```python
from build123d import *

# Parameters (mm, degrees)
SKETCH4_W           = 17
SKETCH4_H           = 67
BOSS_EXTRUDE1_DEPTH = 19.5
FILLET1_R           = 1.5
SKETCH5_W           = 13
SKETCH5_H           = 24.5
CUT_EXTRUDE1_DEPTH  = 17.5
SKETCH6_W           = 5.5
SKETCH6_H           = 5.6
CUT_EXTRUDE2_DEPTH  = 12.7
FILLET2_R           = 1
SKETCH7_R           = 1
CUT_EXTRUDE3_DEPTH  = 337.829426821
SKETCH8_W           = 9.5
SKETCH8_H           = 4.5
CUT_EXTRUDE4_DEPTH  = 5
SKETCH9_W           = 8.343526146
SKETCH9_H           = 4.5
CUT_EXTRUDE5_DEPTH  = 5


with BuildPart() as part:
    # Sketch4 → Boss-Extrude1 (new body)
    with BuildSketch(Plane.XY.offset(30)):
        with Locations((-184.236990356, 242.047210693)):
            Rectangle(SKETCH4_W, SKETCH4_H)
    extrude(amount=BOSS_EXTRUDE1_DEPTH)

    # Fillet1
    fillet1_edges = [part.edges().sort_by_distance(p)[0] for p in [
        (-192.736990356, 275.547210693, 39.75),
        (-175.736990356, 275.547210693, 39.75),
        (-175.736990356, 208.547210693, 39.75),
        (-192.736990356, 208.547210693, 39.75),
    ]]
    fillet(fillet1_edges, radius=FILLET1_R)

    # Sketch5 → Cut-Extrude1 (cut)
    with BuildSketch(Plane.XY.offset(49.5)):
        with Locations((-184.236990356, 259.497210693)):
            Rectangle(SKETCH5_W, SKETCH5_H)
        with Locations((-184.236990356, 225.797210693)):
            Rectangle(SKETCH5_W, SKETCH5_H)
    extrude(amount=-CUT_EXTRUDE1_DEPTH, mode=Mode.SUBTRACT)

    # Sketch6 → Cut-Extrude2 (cut)
    with BuildSketch(Plane.XY.offset(49.5)):
        with Locations((-189.986990356, 242.647210693)):
            Rectangle(SKETCH6_W, SKETCH6_H)
        with Locations((-178.486990356, 242.647210693)):
            Rectangle(SKETCH6_W, SKETCH6_H)
    extrude(amount=-CUT_EXTRUDE2_DEPTH, mode=Mode.SUBTRACT)

    # Fillet2
    fillet2_edges = [part.edges().sort_by_distance(p)[0] for p in [
        (-192.736990356, 239.847210693, 43.15),
        (-192.736990356, 245.447210693, 43.15),
        (-175.736990356, 245.447210693, 43.15),
        (-175.736990356, 239.847210693, 43.15),
    ]]
    fillet(fillet2_edges, radius=FILLET2_R)

    # Sketch7 → Cut-Extrude3 (cut, through all)
    with BuildSketch(Plane.XY.offset(49.5)):
        with Locations((-184.236990356, 273.547210693)):
            Circle(SKETCH7_R)
        with Locations((-184.236990356, 210.747210693)):
            Circle(SKETCH7_R)
        with Locations((-184.236990356, 245.247210693)):
            Circle(SKETCH7_R)
        with Locations((-184.236990356, 239.247210693)):
            Circle(SKETCH7_R)
    extrude(amount=-CUT_EXTRUDE3_DEPTH, mode=Mode.SUBTRACT)

    # Sketch8 → Cut-Extrude4 (cut)
    with BuildSketch(Plane(origin=(0, 208.547210693, 0), x_dir=(-1, 0, 0), z_dir=(0, -1, 0))):
        with Locations((184.186990356, -34.25)):
            Rectangle(SKETCH8_W, SKETCH8_H)
    extrude(amount=-CUT_EXTRUDE4_DEPTH, mode=Mode.SUBTRACT)

    # Sketch9 → Cut-Extrude5 (cut)
    with BuildSketch(Plane(origin=(0, 275.547210693, 0), x_dir=(1, 0, 0), z_dir=(0, 1, 0))):
        with Locations((-183.608753429, -34.25)):
            Rectangle(SKETCH9_W, SKETCH9_H)
    extrude(amount=-CUT_EXTRUDE5_DEPTH, mode=Mode.SUBTRACT)


solid = part.part
```
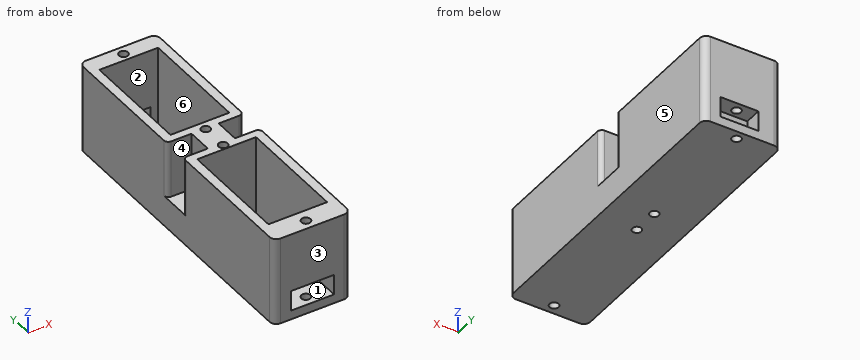
Source: CAD feature listing. Evaluate the final solid. Frame: model axes, mm. Face numbers are marked on the shaded views. A direction names the side the tool comes from. Give positions to 0.01 mm unless a question says otherwise; leave off trailing zeros. Order: outer loops, then holes, each group sorted by start corner. A loop starts at its lowest first (then second) coordinate and runs counter-clockwise, first axis right, second up.
(1) Contact query for flat-ended pins moving along their axis: P1, Ø2.5, axis at x = -184.24, y = 273.55, coming from the -Z side; P2, Ø6.5, axis at x = -182.5, y = 230.5, coming from the +Z side. Output: stop coordinate, or through.
(2) Section query C-C (y = 256). Return the cut outline in (x, z).
(3) Pull-direction query (X, two-part tool) for the marked faces 4, 5 and 6; classes: +X half, -X half, draft (parallel to the pull), parting line (faces both ways), or undercut.
(4) Section query B-B (z = 35.25). Return the cut outline in (x, y).
(5) Access query for the marked faces 1, 2 and 3. Directions: +Z, -Z, +X, -X, +Y, -Y. A direction counts if a zero-diameter tool reaches every point of the face in a straight line with its end or side. Return the directions, or none.
(6) Material intervals for line 1 along Y through (x, z) = (-178.75, 47); line 2 along Y through (x, z) = (-185.75, 40.75); line 3 along Y through (x, z) = (-184.25, 35.75), sorted ascending.
(7) Section query A-A (x = -186.5). Return the cut outline in (y, z), plus the area to 3 significant figures.
(8) Section query D-D (z = 42). State how many separate pieces and enclosed holes the cut face has, plus the area to 3 significant figures.
Outcome:
1. P1: stops at z = 30
1. P2: stops at z = 32
2. outline: (-192.74, 30) - (-175.74, 30) - (-175.74, 49.5) - (-177.74, 49.5) - (-177.74, 32) - (-190.74, 32) - (-190.74, 49.5) - (-192.74, 49.5) - close
3. face 4: draft
3. face 5: +X half
3. face 6: undercut
4. outline: (-192.74, 210.05) arc R1.5 ccw to (-191.24, 208.55) - (-188.94, 208.55) - (-188.94, 213.55) - (-190.74, 213.55) - (-190.74, 238.05) - (-177.74, 238.05) - (-177.74, 213.55) - (-179.44, 213.55) - (-179.44, 208.55) - (-177.24, 208.55) arc R1.5 ccw to (-175.74, 210.05) - (-175.74, 274.05) arc R1.5 ccw to (-177.24, 275.55) - (-179.44, 275.55) - (-179.44, 271.75) - (-177.74, 271.75) - (-177.74, 247.25) - (-190.74, 247.25) - (-190.74, 271.75) - (-187.78, 271.75) - (-187.78, 275.55) - (-191.24, 275.55) arc R1.5 ccw to (-192.74, 274.05) - close; hole circle Ø2 at (-184.24, 239.25); hole circle Ø2 at (-184.24, 245.25)
5. face 1: none
5. face 2: +Z
5. face 3: +Z, -Z, +X, -X, -Y
6. line 1: y = 208.55 to 213.55, 238.05 to 239.85, 245.45 to 247.25, 271.75 to 275.55
6. line 2: y = 208.55 to 213.55, 238.05 to 247.25, 271.75 to 275.55
6. line 3: y = 238.05 to 238.25, 240.25 to 244.25, 246.25 to 247.25
7. outline: (208.55, 30) - (275.55, 30) - (275.55, 32) - (247.25, 32) - (247.25, 49.5) - (238.05, 49.5) - (238.05, 32) - (208.55, 32) - close; (208.55, 36.5) - (213.55, 36.5) - (213.55, 49.5) - (208.55, 49.5) - close; (271.75, 36.5) - (275.55, 36.5) - (275.55, 49.5) - (271.75, 49.5) - close
7. area: 409 mm2
8. separate pieces: 1
8. enclosed holes: 6
8. area: 425 mm2
